Read the model definition and answer for the solid it produces. Units are mm, in the model's axes. Coordinates: 2 decimals unless noted, no trailing zeros. Write each loop counter-clockwise with the first axis right and the second up, starting at its lowest first coordinate (ties: lowest second). Pieces come first, ordered by that corner, then holes.
1) Find the intervals of material crossed by line 1 (X direction, y = 6, z = 1.5); line 2 (Y direction, x = -4, z = 0.1); line 3 (X direction, y = 9, z = 0.55), in increasing order.
2) The part is cut by section A-A (x = 10). Determine the outline of the cut face in (y, z), then the cut area to 4 significant figures.
3) The part is cut by section B-B (y = 3). Determine the outline of the cut face in (x, z), then the cut area to 4 significant figures.
4) The part is cut by section C-C (z = 0.95). Determine the outline of the cut face in (x, y) (3 decimals), then the cut area to 3 significant figures.
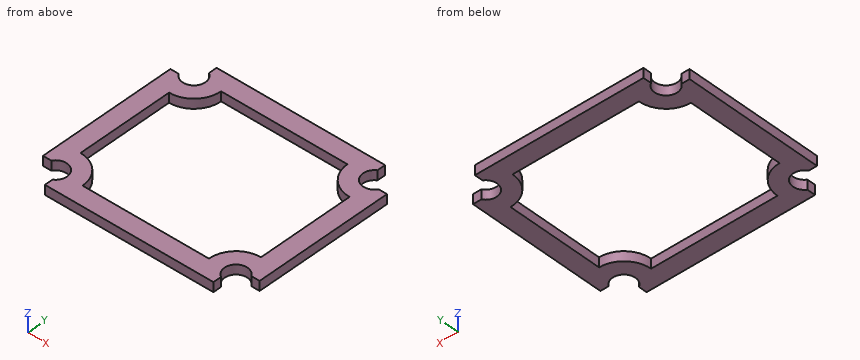
from build123d import *

# Parameters (mm, degrees)
BOSS_EXTRUDE1_DEPTH = 1.5875


with BuildPart() as part:
    # Sketch1 → Boss-Extrude1 (new body)
    with BuildSketch(Plane.XY):
        with BuildLine():
            Line((-18, 11.5), (-18, -11.5))
            Line((-18, -11.5), (-16.621426841, -11.5))
            ThreePointArc((-16.621426841, -11.5), (-13.652961582, -11.152961582), (-14, -14.121426841))
            Line((-14, -14.121426841), (-14, -15.5))
            Line((-14, -15.5), (14, -15.5))
            Line((14, -15.5), (14, -14.121426841))
            ThreePointArc((14, -14.121426841), (13.652961582, -11.152961582), (16.621426841, -11.5))
            Line((16.621426841, -11.5), (18, -11.5))
            Line((18, -11.5), (18, 11.5))
            Line((18, 11.5), (16.621426841, 11.5))
            ThreePointArc((16.621426841, 11.5), (13.652961582, 11.152961582), (14, 14.121426841))
            Line((14, 14.121426841), (14, 15.5))
            Line((14, 15.5), (-14, 15.5))
            Line((-14, 15.5), (-14, 14.121426841))
            ThreePointArc((-14, 14.121426841), (-13.652961582, 11.152961582), (-16.621426841, 11.5))
            Line((-16.621426841, 11.5), (-18, 11.5))
        make_face()
        with BuildLine():
            Line((-15, 8), (-15, -8))
            ThreePointArc((-15, -8), (-11.818019485, -9.318019485), (-10.5, -12.5))
            Line((-10.5, -12.5), (10.5, -12.5))
            ThreePointArc((10.5, -12.5), (11.818019485, -9.318019485), (15, -8))
            Line((15, -8), (15, 8))
            ThreePointArc((15, 8), (11.818019485, 9.318019485), (10.5, 12.5))
            Line((10.5, 12.5), (-10.5, 12.5))
            ThreePointArc((-10.5, 12.5), (-11.818019485, 9.318019485), (-15, 8))
        make_face(mode=Mode.SUBTRACT)
    extrude(amount=BOSS_EXTRUDE1_DEPTH)


solid = part.part
Reported:
1. line 1: x = -18 to -15, 15 to 18
1. line 2: y = -15.5 to -12.5, 12.5 to 15.5
1. line 3: x = -18 to -12.17, 12.17 to 18
2. outline: (-15.5, 0) - (-12.5, 0) - (-12.5, 1.59) - (-15.5, 1.59) - close; (12.5, 0) - (15.5, 0) - (15.5, 1.59) - (12.5, 1.59) - close
2. area: 9.525 mm2
3. outline: (-18, 0) - (-15, 0) - (-15, 1.59) - (-18, 1.59) - close; (15, 0) - (18, 0) - (18, 1.59) - (15, 1.59) - close
3. area: 9.525 mm2
4. outline: (-18, -11.5) - (-16.621, -11.5) arc R1.905 cw (long way) to (-14, -14.121) - (-14, -15.5) - (14, -15.5) - (14, -14.121) arc R1.905 cw (long way) to (16.621, -11.5) - (18, -11.5) - (18, 11.5) - (16.621, 11.5) arc R1.905 cw (long way) to (14, 14.121) - (14, 15.5) - (-14, 15.5) - (-14, 14.121) arc R1.905 cw (long way) to (-16.621, 11.5) - (-18, 11.5) - close; hole (-15, -8) arc R4.5 cw to (-10.5, -12.5) - (10.5, -12.5) arc R4.5 cw to (15, -8) - (15, 8) arc R4.5 cw to (10.5, 12.5) - (-10.5, 12.5) arc R4.5 cw to (-15, 8) - close
4. area: 350 mm2
